Geometry: final body of the model. Coordinates: model frame, mm. A direction names the side the tool comes from. Round coordinates to 2 decimals unless told otherwise and drop trailing zeros. Loops run counter-clockwise (first coordinate to the right, second up) from the corner with the lowest first, then second, coordinate; pieces in that order, holes last. Notation, with made-up numbers: M 89.5,6 L 147.5,6 A26 cw 147.5,26 Z; hole C 28,-20 d9. An arc over 180 degrees is marked long. Answer as a JSON object with one key per item and string values.
from build123d import *

# Parameters (mm, degrees)
SKETCH_1_R          = 1.55
SKETCH_1_W          = 14.95
SKETCH_1_H          = 4.95
EXTRUDE_1_DEPTH     = 2.5
SKETCH_2_R          = 0.75
CUT_EXTRUDE_1_DEPTH = 6
CHAMFER_1_SIZE      = 2


with BuildPart() as part:
    # 草图1 → 凸台-拉伸1 (new body, symmetric)
    with BuildSketch(Plane.XY):
        Polygon((-16, -2.5), (-16, -9.5), (16, -9.5), (16, -2.5), (12.5, -2.5), (12.5, 9.5), (-12.5, 9.5), (-12.5, -2.5), align=None)
        with Locations((-12.5, -6)):
            Circle(SKETCH_1_R, mode=Mode.SUBTRACT)
        with Locations((12.5, -6)):
            Circle(SKETCH_1_R, mode=Mode.SUBTRACT)
        with Locations((0, 6)):
            Circle(SKETCH_1_R, mode=Mode.SUBTRACT)
        Rectangle(SKETCH_1_W, SKETCH_1_H, mode=Mode.SUBTRACT)
    extrude(amount=EXTRUDE_1_DEPTH, both=True)

    # 草图2 → 切除-拉伸1 (cut, through all)
    with BuildSketch(Plane.XY.offset(2.5)):
        with Locations((-13.25, -2.5)):
            Circle(SKETCH_2_R)
        with Locations((-6.725, -2.475)):
            Circle(SKETCH_2_R)
        with Locations((-6.725, 2.475)):
            Circle(SKETCH_2_R)
        with Locations((6.725, 2.475)):
            Circle(SKETCH_2_R)
        with Locations((6.725, -2.475)):
            Circle(SKETCH_2_R)
        with Locations((13.25, -2.5)):
            Circle(SKETCH_2_R)
    extrude(amount=-CUT_EXTRUDE_1_DEPTH, mode=Mode.SUBTRACT)

    # 倒角1
    chamfer_1_edges = [part.edges().sort_by_distance(p)[0] for p in [
        (-16, -9.5, 0),
        (-12.5, 9.5, 0),
        (12.5, 9.5, 0),
        (16, -9.5, 0),
    ]]
    chamfer(chamfer_1_edges, length=CHAMFER_1_SIZE)


solid = part.part
1) Reachability of faces 1 (the cylindrical face through (-6.741, -3.225, 0.035)), 2 (the cylindrical face through (13.23, -3.25, 0.04)), 3 (the flat face through (-15, -2.5, 0)) from +Z, -Z, +X, -X, +Y, -Y: full face, straight path, thin tool, end or side. Return the list, or none.
Results:
{"face 1": "+Z, -Z", "face 2": "+Z, -Z, +Y", "face 3": "+Z, -Z, -X, +Y"}
2) Section query A-A (y = -6). Return the cut outline in (x, z), and give its area (3 significant figures).
Results:
{"outline": "M -16,-2.5 L -14.05,-2.5 L -14.05,2.5 L -16,2.5 Z; M -10.95,-2.5 L 10.95,-2.5 L 10.95,2.5 L -10.95,2.5 Z; M 14.05,-2.5 L 16,-2.5 L 16,2.5 L 14.05,2.5 Z", "area": "129 mm2"}
3) Pin query (flat end, axial travel): P1, Ø0.6, axis at x = 15.5, z = -0.5, coming from the +Y side; P2, Ø2.5, axis at y = 0, z = 1, coming from the +X side; P3, Ø2.5, axis at y = 2, z = 1, coming from the -X side. Return the tip coordinate at first contact, or that it passes through.
Results:
{"P1": "y = -2.5", "P2": "x = 12.5", "P3": "x = -12.5"}
4) Pull-direction query (Z, two-part tool) for faces 4 (the flat face through (0, -4, 2.5)), 5 (the flat face through (0, -4, -2.5)), 6 (the cylindrical face through (6.709, -3.225, 0.035)); classes: +Z half, -Z half, draft (parallel to the pull), parting line (faces both ways), or undercut.
Results:
{"face 4": "+Z half", "face 5": "-Z half", "face 6": "draft"}
5) Ray query, line 1 (Y direction, x = -2.5, z = 0.55) (3 decimals); line 2 (X direction, y = 2.75, z = -0.2); line 3 (Y direction, x = 0, z = 1.7) (3 decimals). Return the intervals inside material, ascending.
Results:
{"line 1": "-9.5 to -2.475, 2.475 to 9.5", "line 2": "-12.5 to -7.42, -6.03 to 6.03, 7.42 to 12.5", "line 3": "-9.5 to -2.475, 2.475 to 4.45, 7.55 to 9.5"}
6) Section query B-B (z = 1.15). Return the cut outline in (x, y) (3 decimals).
Results:
{"outline": "M -16,-7.5 L -14,-9.5 L 14,-9.5 L 16,-7.5 L 16,-2.5 L 14,-2.5 A0.75 cw 12.5,-2.5 L 12.5,7.5 L 10.5,9.5 L -10.5,9.5 L -12.5,7.5 L -12.5,-2.5 A0.75 cw -14,-2.5 L -16,-2.5 Z; hole C -12.5,-6 d3.1; hole M -7.475,-2.475 A0.75 ccw -5.975,-2.475 L 5.975,-2.475 A0.75 ccw 7.475,-2.475 L 7.475,2.475 A0.75 ccw 5.975,2.475 L -5.975,2.475 A0.75 ccw -7.475,2.475 Z; hole C 0,6 d3.1; hole C 12.5,-6 d3.1"}
7) Section query D-D (x = -1). Return the cut outline in (y, z) (3 decimals), and give its area (3 significant figures).
Results:
{"outline": "M -9.5,-2.5 L -2.475,-2.5 L -2.475,2.5 L -9.5,2.5 Z; M 2.475,-2.5 L 4.816,-2.5 L 4.816,2.5 L 2.475,2.5 Z; M 7.184,-2.5 L 9.5,-2.5 L 9.5,2.5 L 7.184,2.5 Z", "area": "58.4 mm2"}
8) Section query C-C (y = 1.25). Return the cut outline in (x, z) (3 decimals), and give its area (4 significant figures).
Results:
{"outline": "M -12.5,-2.5 L -7.475,-2.5 L -7.475,2.5 L -12.5,2.5 Z; M 7.475,-2.5 L 12.5,-2.5 L 12.5,2.5 L 7.475,2.5 Z", "area": "50.25 mm2"}
